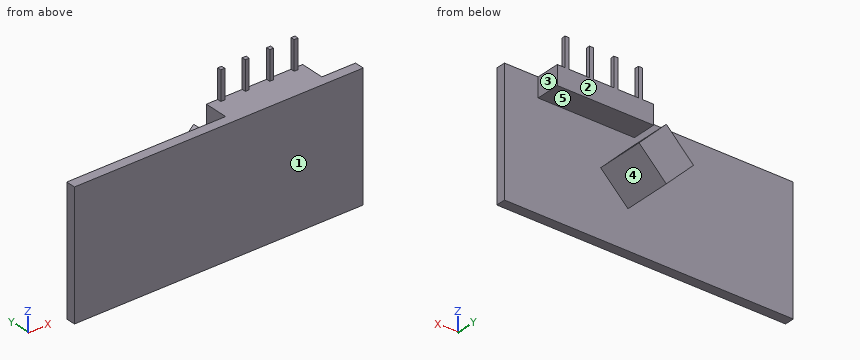
```python
from build123d import *

# Parameters (mm, degrees)
SKETCH1_W           = 30
SKETCH1_H           = 13
BOSS_EXTRUDE1_DEPTH = 1
SKETCH2_W           = 10
SKETCH2_H           = 2
BOSS_EXTRUDE2_DEPTH = 2.5
SKETCH4_W           = 0.4064
SKETCH4_H           = 0.4064
BOSS_EXTRUDE3_DEPTH = 3
LPATTERN1_COUNT     = 4
LPATTERN1_PITCH     = 2.54
BOSS_EXTRUDE4_DEPTH = 5


with BuildPart() as part:
    # Sketch1 → Boss-Extrude1 (new body)
    with BuildSketch(Plane(origin=(0, 0, 0), x_dir=(1, 0, 0), z_dir=(0, 1, 0))):
        Rectangle(SKETCH1_W, SKETCH1_H)
    extrude(amount=BOSS_EXTRUDE1_DEPTH)

    # Sketch2 → Boss-Extrude2 (add)
    with BuildSketch(Plane(origin=(0, 1, 0), x_dir=(1, 0, 0), z_dir=(0, 1, 0))):
        with Locations((6.5, -5.5)):
            Rectangle(SKETCH2_W, SKETCH2_H)
    extrude(amount=BOSS_EXTRUDE2_DEPTH)

    # Sketch4 → Boss-Extrude3 (add)
    with BuildSketch(Plane.XY.offset(6.5)):
        with Locations((10.5, 3.2968)):
            Rectangle(SKETCH4_W, SKETCH4_H)
    boss_extrude3 = extrude(amount=BOSS_EXTRUDE3_DEPTH)

    # LPattern1: Boss-Extrude3 ×4
    with Locations(*[(-i * LPATTERN1_PITCH, 0, 0) for i in range(1, LPATTERN1_COUNT)]):
        add(boss_extrude3)

    # Sketch5 → Boss-Extrude4 (add)
    with BuildSketch(Plane(origin=(0, 1, 0), x_dir=(1, 0, 0), z_dir=(0, 1, 0))):
        Polygon((-0.656854249, -0.328427125), (2.171572875, -3.156854249), (5, -0.328427125), (2.171572875, 2.5), align=None)
    extrude(amount=BOSS_EXTRUDE4_DEPTH)


solid = part.part
```
The model under review builds one solid part; all positions refer to its coordinate system, in mm. Face numbers are marked on the shaded views. A direction names the side the tool comes from. Give positions to 0.01 mm unless a question says otherwise; leave off trailing zeros. Order: outer loops, then holes, each group sorted by start corner. A loop starts at its lowest first (then second) coordinate and runs counter-clockwise, first axis right, second up. Notation, with made-up numbers: (77.5, 18.5) - (123.5, 18.5) arc R27 ccw to (123.5, 51.5) - close; hole circle Ø6 at (-27, -26.75). An arc over 180 degrees is marked (long way). Use CSV: the item, a comma, the result in double quotes. Start each with the question number.
Q1. We need section D-D, the plane z = -0.5. Write out the cut boundary in (x, y), and give its area (3 significant figures).
Q2. We need section B-B, the plane y = 2.1. Write out the cut boundary in (x, z).
Q3. We need section C-C, the plane x = -3.25. Write out the cut boundary in (y, z).
Q4. We need section A-A, the plane z = 8.25. Write out the cut boundary in (x, y).
Q5. To check wall thickness, follow line 1 along Y through (x, z) = (-5.75, 1.5); line 2 along Y through (x, z) = (5.75, 5); line 3 along Z through (x, y) = (4.75, 2.6). State the ranges of each line that lie inside material, in increasing order. Write a range as [from, to].
Q6. The part is to be moulded in two halves that separate along Z. For the marked faces 3, 4 and 5, say which applies: +Z half, -Z half, draft (parallel to the pull), parting line (faces both ways), or undercut.
Q7. Clearance check with flat-ended pins moving along their axes: pin 1 Ø2 at (y, z) = (3.5, 3.5) entering from -X; pin 2 Ø1 at (x, y) = (3.5, 4.5) entering from -Z; pin 3 Ø1 at (y, z) = (5, -0.5) entering from +X; pin 4 Ø2 at (y, z) = (1.5, 8) entering from -X. State where each tip first meets the part, or that it passes through.
Q8. Tool access review of the marked faces 1 and 2: name each direction out of +Z, -Z, +X, -X, +Y, -Y from which nothing blocks a thin tool from reaching the whole face with its end or side.
Outcome:
1,outline,"(-15, 0) - (15, 0) - (15, 1) - (4.17, 1) - (4.17, 6) - (0.17, 6) - (0.17, 1) - (-15, 1) - close"
1,area,"50.0 mm^2"
2,outline,"(-0.66, 0.33) - (2.17, -2.5) - (5, 0.33) - (2.17, 3.16) - close; (1.5, 4.5) - (11.5, 4.5) - (11.5, 6.5) - (1.5, 6.5) - close"
3,outline,"(0, -6.5) - (1, -6.5) - (1, 6.5) - (0, 6.5) - close"
4,outline,"(2.68, 3.09) - (3.08, 3.09) - (3.08, 3.5) - (2.68, 3.5) - close; (5.22, 3.09) - (5.62, 3.09) - (5.62, 3.5) - (5.22, 3.5) - close; (7.76, 3.09) - (8.16, 3.09) - (8.16, 3.5) - (7.76, 3.5) - close; (10.3, 3.09) - (10.7, 3.09) - (10.7, 3.5) - (10.3, 3.5) - close"
5,line 1,"y = [0, 1]"
5,line 2,"y = [0, 3.5]"
5,line 3,"z = [0.08, 0.58], [4.5, 6.5]"
6,face 3,"draft"
6,face 4,"-Z half"
6,face 5,"undercut"
7,pin 1,"stops at x = 1.51"
7,pin 2,"stops at z = -1.67"
7,pin 3,"stops at x = 4.67"
7,pin 4,"passes through"
8,face 1,"+Z, -Z, +X, -X, -Y"
8,face 2,"+Z, +X, -X, +Y"
